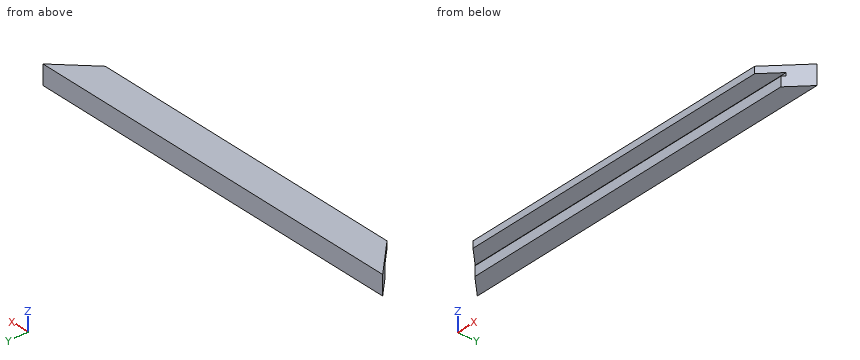
```python
from build123d import *

# Parameters (mm, degrees)
F1_DEPTH = 205
F3_DEPTH = 25.4


with BuildPart() as f1:
    # F0 (on Right) → F1 (new body, symmetric)
    with BuildSketch(Plane.YZ):
        Polygon((17.2946, -10), (17.2946, 10.3), (-17.7054, 10.3), (-17.7054, 3.3), (0, 3.3), (0, 0), (-3, 0), (-3, -10), align=None)
    extrude(amount=F1_DEPTH, both=True)

    # F2 (on face) → F3 (cut)
    with BuildSketch(Plane.XY.offset(10.3)):
        Polygon((-170, -17.7054), (-205, 17.2946), (-205, -17.7054), align=None)
        Polygon((205, -17.7054), (205, 17.2946), (170, -17.7054), align=None)
    extrude(amount=-F3_DEPTH, mode=Mode.SUBTRACT)


solid = f1.part
```
Part model, mm, in its own coordinate system. Round coordinates to 2 decimals unless told otherwise and drop trailing zeros. Write each loop counter-clockwise with the first axis right and the second up, starting at its lowest first coordinate (ties: lowest second). Pieces come first, ordered by that corner, then holes. Notation, with made-up numbers: (14.5, 48.25) -> (22.5, 48.25) arc R18 cw to (22.5, 78.25) -> close; hole circle Ø2 at (21, 79.5). An arc over 180 degrees is marked (long way). Return JSON: item names as keys, results as strings. Group by question number.
Q1. Saw through at C-C on y = 6. Write the cut outline in (x, z).
Q2. Saw through at B-B on z = -4. Write the cut outline in (x, y), plus the area to 3 significant figures.
Q3. Probe L1, parallel to Z at x = -26.5, y = -1; L2, parallel to Z at x = -124.5, y = -12.5; L3, parallel to Y at x = -99.5, z = 2.5. List the from-to ranges inside material, lowest first. Write a range as [from, to].
Q4. Pin check, flat tips, straight feed: pin 1 (6 mm diameter, centred on y = 13.5, z = 0, fed in from -X); pin 2 (2 mm diameter, centred on y = 7.5, z = -3.5, fed in from -X); pin 3 (5 mm diameter, centred on x = 144.5, y = -3.5, fed in from -Z); pin 4 (6 mm diameter, centred on y = -9, z = 5.5, fed in from -X). Stop position of each tip, or through.
Q5. Saw through at A-A on x = -28. Write the cut outline in (y, z), plus the area to 3 significant figures.
Answer:
{
 "1": {"outline": "(-193.71, -10) -> (193.71, -10) -> (193.71, 10.3) -> (-193.71, 10.3) -> close"},
 "2": {"outline": "(-205, 17.29) -> (-184.71, -3) -> (184.71, -3) -> (205, 17.29) -> close", "area": "7,910 mm2"},
 "3": {"L1": "[-10, 0], [3.3, 10.3]", "L2": "[3.3, 10.3]", "L3": "[0, 17.29]"},
 "4": {"pin 1": "x = -204.21", "pin 2": "x = -196.21", "pin 3": "z = -10", "pin 4": "x = -181.71"},
 "5": {"outline": "(-17.71, 3.3) -> (0, 3.3) -> (0, 0) -> (-3, 0) -> (-3, -10) -> (17.29, -10) -> (17.29, 10.3) -> (-17.71, 10.3) -> close", "area": "505 mm2"}
}
